Verification items for the finished model (mm, model axes). A direction names the side the tool comes from. Round coordinates to 2 decimals unless told otherwise and drop trailing zeros. Order: outer loops, then holes, each group sorted by start corner. A loop starts at its lowest first (then second) coordinate and runs counter-clockwise, first axis right, second up.
```python
from build123d import *

# Parameters (mm, degrees)
SKETCH002_R     = 1.65
PAD002_DEPTH    = 12.5
SKETCH003_R     = 1.75
PAD003_DEPTH    = 7
SKETCH004_W     = 10.021474
SKETCH004_H     = 5.992485
POCKET_DEPTH    = 10
SKETCH005_R     = 1.6
POCKET001_DEPTH = 30
FILLET001_R     = 1


with BuildPart() as part:
    # Sketch002 → Pad002 (new body)
    with BuildSketch(Plane.XY):
        with BuildLine():
            Line((5.4, 0), (22.4, 0))
            Line((22.4, 0), (22.4, 4))
            Line((22.4, 4), (27.6, 4))
            Line((27.6, 4), (27.6, 31))
            Line((27.6, 31), (1.7, 31))
            Line((1.7, 25.6), (1.7, 31))
            Line((0, 25.6), (1.7, 25.6))
            Line((0, 25.6), (0, 5.4))
            ThreePointArc((5.4, 0), (3.818377, 3.818377), (0, 5.4))
        make_face()
        with Locations((12.4, 25.5)):
            Circle(SKETCH002_R, mode=Mode.SUBTRACT)
        with Locations((12.4, 5.5)):
            Circle(SKETCH002_R, mode=Mode.SUBTRACT)
    extrude(amount=PAD002_DEPTH)

    # Sketch003 (on Face5 of Pad002) → Pad003 (join)
    with BuildSketch(Plane(origin=(0, 31, 0), x_dir=(-1, 0, 0), z_dir=(0, 1, 0))):
        with BuildLine():
            Line((-27.6, 0), (-21.8, 0))
            Line((-21.8, 0), (-21.8, 4.5))
            ThreePointArc((-21.8, 4.5), (-24.7, 7.4), (-27.6, 4.5))
            Line((-27.6, 4.5), (-27.6, 0))
        make_face()
        with Locations((-24.7, 4.5)):
            Circle(SKETCH003_R, mode=Mode.SUBTRACT)
    extrude(amount=PAD003_DEPTH)

    # Sketch004 (on Face6 of Pad003) → Pocket (cut)
    with BuildSketch(Plane(origin=(0, 0, 0), x_dir=(0, -1, 0), z_dir=(-1, 0, 0))):
        with Locations((-15.491406, 3.567648)):
            Rectangle(SKETCH004_W, SKETCH004_H)
    extrude(amount=-POCKET_DEPTH, mode=Mode.SUBTRACT)

    # Sketch005 (on Face7 of Pocket) → Pocket001 (cut)
    with BuildSketch(Plane.XZ.offset(-4)):
        with Locations((24.7, 4.5)):
            Circle(SKETCH005_R)
    extrude(amount=-POCKET001_DEPTH, mode=Mode.SUBTRACT)

    # Fillet001
    fillet001_edges = [part.edges().sort_by_distance(p)[0] for p in [
        (23.1, 4, 4.5),
    ]]
    fillet(fillet001_edges, radius=FILLET001_R)


with BuildPart() as part_1:
    # Body001 placement: moved
    add(part.part.moved(Location((20.4, 0, 4))))


solid = part_1.part
```
1) Tool access check on faces 1 (the flat face through (42.8, 2, 10)), 2 (the flat face through (21, 25.6, 10)), 3 (the flat face through (25, 16, 4.571)), 4 (the cylindrical face through (45, 34.5, 11.4)). Record the directions out of +Z, -Z, +X, -X, +Y, -Y that give a thin tool (end or side, any length) a straight path to the whole face; none if there is none.
2) Sectioned sample at D-D on x = 45.1. Record the cut outline in (y, z), then the cut area to 3 significant figures.
3) Go/stop test with flat-tipped pins: pin 1 Ø1.6 at (x, z) = (45.5, 7.5) entering from -Y; pin 2 Ø3 at (y, z) = (16.5, 7) entering from -X; pin 3 Ø4 at (x, z) = (30.5, 12.5) entering from +Y. Record where each tip stops, or that it passes through.
4) Sectioned sample at C-C on x = 27.75. Record the cut outline in (y, z).
5) Scan lines: probe 1 along Y at (x, z) = (32.8, 13); probe 2 along Y at (x, z) = (26.75, 9); probe 3 along Z at (x, y) = (30, 15). Record each from-to range of solid material in increasing order.
6) Sectioned sample at A-A on x = 32.8. Record the cut outline in (y, z).
7) Sectioned sample at B-B on y = 32. Record the cut outline in (x, z), then the cut area to 3 significant figures.
8) Draft check along Z on faces 5 (the flat face through (25, 20.502, 8)), 6 (the flat face through (20.4, 16, 12)), 7 (the flat face through (34, 16, 16.5)). Enter one of: released by +Z, released by -Z, zero draft, split by the parting line, or undercut.
Returned:
1. face 1: +Z, -Z, +X, -Y
1. face 2: +Z, -Z, -X, +Y
1. face 3: -X
1. face 4: +Z, +Y
2. outline: (4, 4) - (38, 4) - (38, 6.75) - (31, 6.75) - (31, 6.9) - (5, 6.9) arc R1 ccw to (4, 5.9) - close; (4, 11.1) arc R1 ccw to (5, 10.1) - (31, 10.1) - (31, 10.25) - (38, 10.25) - (38, 11.4) - (31, 11.4) - (31, 16.5) - (4, 16.5) - close
2. area: 278 mm2
3. pin 1: stops at y = 4.31
3. pin 2: stops at x = 30.4
3. pin 3: stops at y = 31
4. outline: (0, 4) - (31, 4) - (31, 16.5) - (0, 16.5) - close; hole (10.48, 4.57) - (20.5, 4.57) - (20.5, 10.56) - (10.48, 10.56) - close
5. probe 1: y = 0 to 3.85, 7.15 to 23.85, 27.15 to 31
5. probe 2: y = 0 to 10.48, 20.5 to 31
5. probe 3: z = 4 to 4.57, 10.56 to 16.5
6. outline: (0, 4) - (3.85, 4) - (3.85, 16.5) - (0, 16.5) - close; (7.15, 4) - (23.85, 4) - (23.85, 16.5) - (7.15, 16.5) - close; (27.15, 4) - (31, 4) - (31, 16.5) - (27.15, 16.5) - close
7. outline: (42.2, 4) - (48, 4) - (48, 8.5) arc R2.9 ccw to (42.2, 8.5) - close; hole circle Ø3.5 at (45.1, 8.5)
7. area: 29.7 mm2
8. face 5: undercut
8. face 6: zero draft
8. face 7: released by +Z
